Read the model definition and answer for the solid it produces. Units are mm, in the model's axes. Face numbers are marked on the shaded views. Coordinates: 2 decimals unless noted, no trailing zeros. Loops run counter-clockwise (first coordinate to the right, second up) from the corner with the lowest first, then second, coordinate; pieces in that order, holes last.
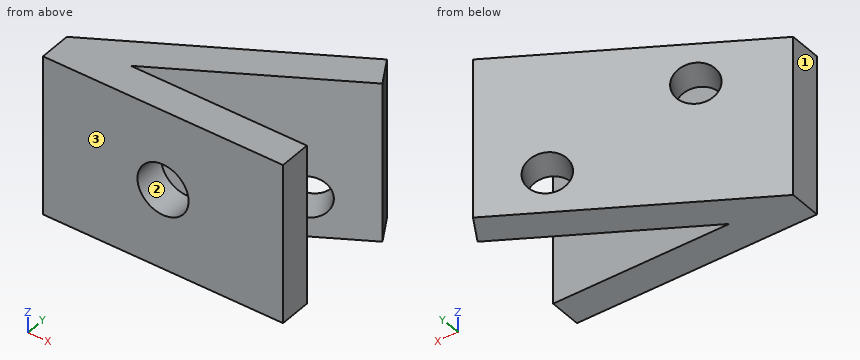
from build123d import *

# Parameters (mm, degrees)
SKETCH2_W           = 15
SKETCH2_H           = 2
BOSS_EXTRUDE1_DEPTH = 10
BOSS_EXTRUDE2_DEPTH = 10
SKETCH4_R           = 1.3
CUT_EXTRUDE1_DEPTH  = 2
SKETCH5_R           = 1.6
CUT_EXTRUDE2_DEPTH  = 2


with BuildPart() as part:
    # Sketch2 → Boss-Extrude1 (new body)
    with BuildSketch(Plane.XY):
        with Locations((7.5, 1)):
            Rectangle(SKETCH2_W, SKETCH2_H)
    extrude(amount=BOSS_EXTRUDE1_DEPTH)

    # Sketch3 → Boss-Extrude2 (add)
    with BuildSketch(Plane.XY.offset(10)):
        Polygon((0, 2), (4, 2), (15, 8.350852961), (14, 10.082903769), align=None)
    extrude(amount=-BOSS_EXTRUDE2_DEPTH)

    # Sketch4 → Cut-Extrude1 (cut)
    with BuildSketch(Plane(origin=(-0.866025404, 1.5, 0), x_dir=(0.8660254037844378, 0.5000000000000016, 0), z_dir=(-0.5000000000000016, 0.8660254037844378, 0))):
        with Locations(Location((5.915807537, -7.5, 0), (0, 0, 180))):
            Circle(SKETCH4_R)
        with Locations(Location((13.415807537, -2.5, 0), (0, 0, 180))):
            Circle(SKETCH4_R)
    extrude(amount=-CUT_EXTRUDE1_DEPTH, mode=Mode.SUBTRACT)

    # Sketch5 → Cut-Extrude2 (cut)
    with BuildSketch(Plane(origin=(0, 2, 0), x_dir=(1, 0, 0), z_dir=(0, 1, 0))):
        with Locations(Location((7.5, -5, 0), (0, 0, 270))):
            Circle(SKETCH5_R)
    extrude(amount=-CUT_EXTRUDE2_DEPTH, mode=Mode.SUBTRACT)


solid = part.part
Q1. Determine the mould class of the marked faces 1, 2 and 3 for opening direction X: +X half, -X half, draft (parallel to the pull), parting line (faces both ways), or undercut.
Findings below:
face 1: -X half
face 2: undercut
face 3: draft
Q2. Straight lines are drawn through the part: probe 1 along X at (y, z) = (1.05, 5); probe 2 along Y at (x, z) = (8.5, 7); probe 3 along Y at (x, z) = (10, 6.5). For each, find the intervals that lie inside material, in ascending order.
Findings below:
probe 1: x = 0 to 5.9, 9.1 to 15
probe 2: y = 0 to 2, 4.6 to 6.91
probe 3: y = 0 to 2, 5.46 to 7.77
Q3. A cutting plane is placed at A-A (z = 5). Give the vertices of the cut face in (x, y).
Findings below:
outline: (0, 0) - (5.9, 0) - (5.9, 2) - (4, 2) - (15, 8.35) - (14, 10.08) - (0, 2) - close; (9.1, 0) - (15, 0) - (15, 2) - (9.1, 2) - close
Q4. A cutting plane is placed at B-B (x = 7.5). Give the vertices of the cut face in (y, z).
Findings below:
outline: (0, 0) - (2, 0) - (2, 3.4) - (0, 3.4) - close; (0, 6.6) - (2, 6.6) - (2, 10) - (0, 10) - close; (4.02, 0) - (6.33, 0) - (6.33, 10) - (4.02, 10) - close
Q5. Flat-ended cylindrical pins translate along their axes: pin 1 Ø6 at (y, z) = (7, 8.5) entering from -X; pin 2 Ø5 at (y, z) = (5, 7.5) entering from -X; pin 3 Ø1 at (x, z) = (2, 1.5) entering from +Y. Find the tip coordinate at first contact, or state that the pin passes through.
Findings below:
pin 1: stops at x = 3.46
pin 2: stops at x = 0.87
pin 3: stops at y = 3.44
Q6. A cutting plane is placed at C-C (y = 1). Give the vertices of the cut face in (x, z), then the cut area to 3 significant figures.
Findings below:
outline: (0, 0) - (15, 0) - (15, 10) - (0, 10) - close; hole circle Ø3.2 at (7.5, 5)
area: 142 mm2
Q7. A cutting plane is placed at D-D (z = 6). Give the vertices of the cut face in (x, y).
Findings below:
outline: (0, 0) - (6.25, 0) - (6.25, 2) - (4, 2) - (15, 8.35) - (14, 10.08) - (0, 2) - close; (8.75, 0) - (15, 0) - (15, 2) - (8.75, 2) - close
